Can you work these out from the model? Positions are in its coordinate system, mm. Face numbers are marked on the shaded views. A direction names the side the tool comes from. Round coordinates to 2 decimals unless told otherwise and drop trailing zeros. Order: outer loops, then holes, each group sorted by start corner. A loop starts at its lowest first (then second) coordinate and runs counter-clockwise, first axis right, second up. Notation, with made-up numbers: M -1.75,42.25 L 37.25,42.25 A24 ccw 37.25,71.25 Z; hole C 79.25,-4.5 d2. An arc over 180 degrees is marked long. One line per question, with ' | ' between items.
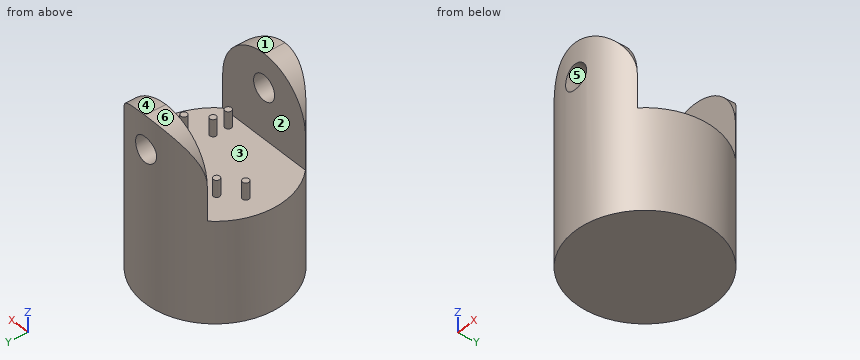
```python
from build123d import *

# Parameters (mm, degrees)
SKETCH1_R               = 4.15
BOSS_EXTRUDE1_DEPTH     = 11
SKETCH2_W               = 8.37511106
SKETCH2_H               = 5.82
CUT_EXTRUDE1_DEPTH      = 5
CUT_EXTRUDE2_DEPTH      = 13.467758419
CUT_EXTRUDE3_DEPTH      = 13.467758574
CUT_EXTRUDE3_DEPTH_BACK = 13.467758574
SKETCH4_R               = 0.75
SKETCH5_R               = 0.19
BOSS_EXTRUDE2_DEPTH     = 1


with BuildPart() as part:
    # Sketch1 → Boss-Extrude1 (new body)
    with BuildSketch(Plane.XY):
        Circle(SKETCH1_R)
    extrude(amount=BOSS_EXTRUDE1_DEPTH)

    # Sketch2 → Cut-Extrude1 (cut)
    with BuildSketch(Plane.XY.offset(11)):
        Rectangle(SKETCH2_W, SKETCH2_H)
    extrude(amount=-CUT_EXTRUDE1_DEPTH, mode=Mode.SUBTRACT)

    # Sketch3 → Cut-Extrude2 (cut, symmetric)
    with BuildSketch(Plane(origin=(0, 0, 0), x_dir=(1, 0, 0), z_dir=(0, 1, 0))):
        with BuildLine():
            Line((-2.958783534, -8.031414478), (-2.958783534, -11))
            Line((-2.958783534, -11), (0, -11))
            ThreePointArc((0, -11), (-2.092768611, -10.127058771), (-2.958783534, -8.031414478))
        make_face()
    cut_extrude2 = extrude(amount=CUT_EXTRUDE2_DEPTH, both=True, mode=Mode.SUBTRACT)

    # Mirror1: Cut-Extrude2 across plane
    add(cut_extrude2.mirror(Plane(origin=(0, 0, 0), x_dir=(0, 0, 1), z_dir=(1, 0, 0))), mode=Mode.SUBTRACT)

    # Sketch4 → Cut-Extrude3 (cut, two sides: drawn at the far end of the back side and taken through both)
    with BuildSketch(Plane(origin=(0, 0, 0), x_dir=(1, 0, 0), z_dir=(0, 1, 0)).offset(-CUT_EXTRUDE3_DEPTH_BACK)):
        with Locations(Location((0, -9, 0), (0, 0, 270))):
            Circle(SKETCH4_R)
    extrude(amount=CUT_EXTRUDE3_DEPTH + CUT_EXTRUDE3_DEPTH_BACK, mode=Mode.SUBTRACT)

    # Sketch5 → Boss-Extrude2 (add)
    with BuildSketch(Plane.XY.offset(6)):
        with Locations((-1.755, 2.26)):
            Circle(SKETCH5_R)
        with Locations((-1.755, 1.36)):
            Circle(SKETCH5_R)
        with Locations((1.755, -1.34)):
            Circle(SKETCH5_R)
        with Locations((1.755, -2.24)):
            Circle(SKETCH5_R)
        with Locations((-2.755, 0.46)):
            Circle(SKETCH5_R)
        with Locations((2.755, -0.44)):
            Circle(SKETCH5_R)
    extrude(amount=BOSS_EXTRUDE2_DEPTH)


solid = part.part
```
(1) Thinking about a two-plate mould opening in X: for the marked faces 4, 5 and 6, which applies, released by +X, released by -X, zero draft, split by the parting line, or undercut?
Final values:
face 4: released by +X | face 5: undercut | face 6: released by -X
(2) If we section it at A-A on z = 6.25: Please give me the cut outline in (x, y) (3 decimals).
Final values:
outline: M -2.959,-2.91 A4.15 ccw 2.959,-2.91 Z; M -2.959,2.91 L 2.959,2.91 A4.15 ccw Z; C -2.755,0.46 d0.38; C -1.755,1.36 d0.38; C -1.755,2.26 d0.38; C 1.755,-2.24 d0.38; C 1.755,-1.34 d0.38; C 2.755,-0.44 d0.38
(3) If we section it at D-D on z = 9.5: Please give me the cut outline in (x, y), plus the area to 3 significant figures.
Final values:
outline: M -2.57,-3.26 A4.15 ccw -0.56,-4.11 L -0.56,-2.91 L -2.57,-2.91 Z; M -2.57,2.91 L -0.56,2.91 L -0.56,4.11 A4.15 ccw -2.57,3.26 Z; M 0.56,-4.11 A4.15 ccw 2.57,-3.26 L 2.57,-2.91 L 0.56,-2.91 Z; M 0.56,2.91 L 2.57,2.91 L 2.57,3.26 A4.15 ccw 0.56,4.11 Z | area: 7.09 mm^2
(4) Please list where these lines run through material, in increasing order: probe 1 along Z at (x, y) = (0, -3); probe 2 along Z at (x, y) = (-3.25, 2); probe 3 along Y at (x, z) = (-2, 7). Write a range as [from, to].
Final values:
probe 1: [0, 8.25], [9.75, 11] | probe 2: [0, 6] | probe 3: [-3.64, -2.91], [2.91, 3.64]
(5) If we section it at B-B on x = -0.25: Please give me the cut outline in (y, z).
Final values:
outline: M -4.14,0 L 4.14,0 L 4.14,8.29 L 2.91,8.29 L 2.91,6 L -2.91,6 L -2.91,8.29 L -4.14,8.29 Z; M -4.14,9.71 L -2.91,9.71 L -2.91,10.99 L -4.14,10.99 Z; M 2.91,9.71 L 4.14,9.71 L 4.14,10.99 L 2.91,10.99 Z
(6) Will these pins go through, and if not, where does the flat tip stop? pin 1 Ø2 at (x, y) = (-2.5, -1) entering from +Z; pin 2 Ø3 at (y, z) = (3, 6.5) entering from +X; pin 3 Ø1.5 at (y, z) = (1.5, 6.5) entering from +X; pin 4 Ø1.4 at (x, z) = (0, 9) entering from +Y.
Final values:
pin 1: z = 6 | pin 2: x = 3.84 | pin 3: x = 4.04 | pin 4: through
(7) If we section it at C-C on y = 2.26: Please give me the cut outline in (x, z) (3 decimals).
Final values:
outline: M -3.481,0 L 3.481,0 L 3.481,6 L -1.565,6 L -1.565,7 L -1.945,7 L -1.945,6 L -3.481,6 Z
(8) On a 3-axis mill with a long thin cutter (end or side, diameter ignored), from which of +Z, -Z, +X, -X, +Y, -Y can I reach the whole of each face in a straight line? I mean the marked faces 1, 2 and 3. Say none if no direction works.
Final values:
face 1: +Z, +X, +Y, -Y | face 2: +Z, +X, -X | face 3: +Z
